The listing builds one solid part. Answer for the finished solid, in the listing's coordinates (mm). Round coordinates to 2 decimals unless told otherwise and drop trailing zeros. Loops run counter-clockwise (first coordinate to the right, second up) from the corner with the lowest first, then second, coordinate; pieces in that order, holes last. Notation, with made-up numbers: M -11,87 L 34,87 A23 cw 34,115 Z; hole C 72,39.25 d11. An arc over 180 degrees is marked long. Put each result on its own line as item: value. Start each with the question number.
(1) Flat-ended cylindrical pins translate along their axes: P1, Ø2, axis at x = -2, z = 24, coming from the -Y side (3 decimals); P2, Ø4, axis at y = -5.5, z = 25.5, coming from the +X side. Find the tip coordinate at first contact, or state that the pin passes through.
(2) Section B-B, the plane z = 28 is taken. Determine the outline of the cut face in (x, y) (3 decimals), then the cut area to 3 significant figures.
(3) Section C-C, the plane x = 1 is taken. Determine the outline of the cut face in (y, z) (3 decimals).
(4) Straight lines are drawn through the part: line 1 (Y direction, x = -1.75, z = 42) (3 decimals); line 2 (Z direction, x = 0.25, y = -8.5); line 3 (Z direction, x = 2, y = -15). For each, find the intervals that lie inside material, in ascending order.
(5) Section A-A, the plane y = -9 is taken. Determine the outline of the cut face in (x, z).
```python
from build123d import *

# Parameters (mm, degrees)
F0_W     = 6.096
F0_H     = 114.3
F1_DEPTH = 3.175
F3_DEPTH = 12.7


with BuildPart() as f1:
    # F0 (on Front) → F1 (new body, symmetric)
    with BuildSketch(Plane.XZ):
        Rectangle(F0_W, F0_H)
    extrude(amount=F1_DEPTH, both=True)

    # F2 (on face) → F3 (join)
    with BuildSketch(Plane.XZ.offset(3.175)):
        with BuildLine():
            ThreePointArc((0, 56.7182), (-1.796051, 52.382149), (2.54, 54.1782))
            ThreePointArc((2.54, 54.1782), (1.796051, 55.974251), (0, 56.7182))
        make_face()
    extrude(amount=F3_DEPTH)


solid = f1.part
```
Recorded:
1. P1: stops at y = -3.175
1. P2: passes through
2. outline: M -3.048,-3.175 L 3.048,-3.175 L 3.048,3.175 L -3.048,3.175 Z
2. area: 38.7 mm²
3. outline: M -15.875,51.843 L -3.175,51.843 L -3.175,-57.15 L 3.175,-57.15 L 3.175,57.15 L -3.175,57.15 L -3.175,56.513 L -15.875,56.513 Z
4. line 1: y = -3.175 to 3.175
4. line 2: z = 51.65 to 56.71
4. line 3: z = 52.61 to 55.74
5. outline: C 0,54.18 d5.08
